Here's the drawing with two shaded views (mm, measured from the low corner). I have some questions. A direction names the side the tool comes from. Give positions to 0.01 mm unless a question says otherwise; leave off trailing zeros. Loops run counter-clockwise (first coordinate to the right, second up) from the corner with the lowest first, then second, coordinate; pieces in that order, holes last. Notation, with made-up numbers: M -2,45.25 L 32,45.25 A18 ccw 32,80.25 Z; hole C 3.25,-13 d5. An arc over 180 degrees is marked long. Write item = value, one per line. Start each with the question number.
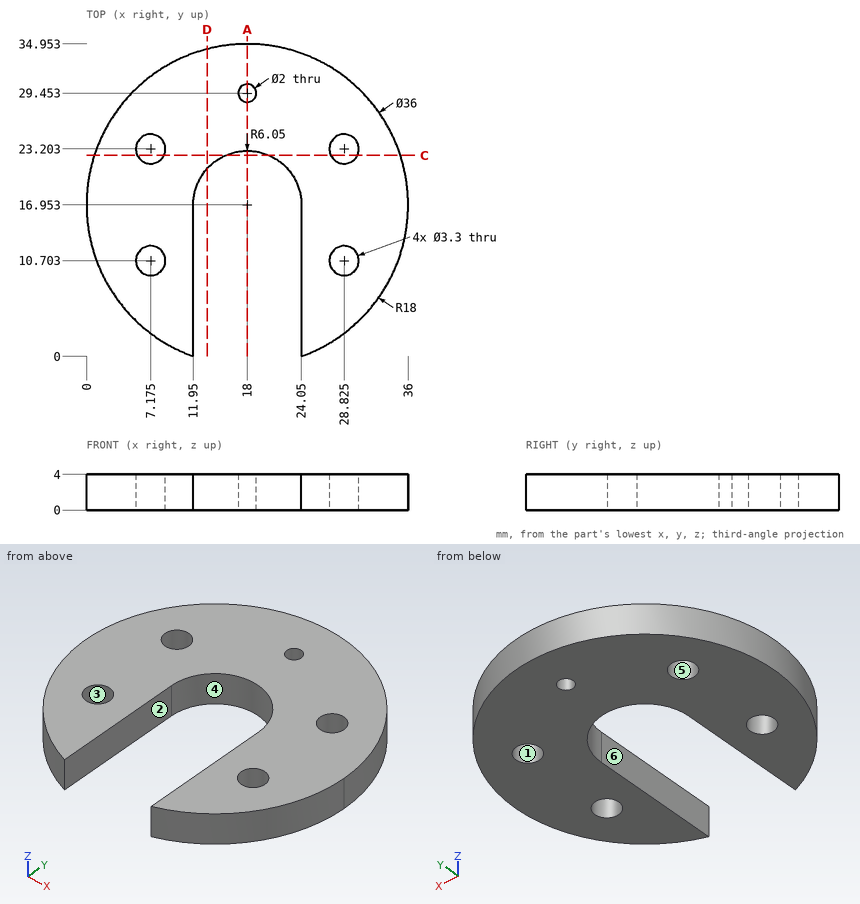
Q1. On a 3-axis mill with a long thin cutter (end or side, diameter ignored), from which of +Z, -Z, +X, -X, +Y, -Y can I reach the whole of each face in a straight line? I mean the marked faces 5 and 6. Say none if no direction works.
Q2. If we section it at D-D, the plane x = 13.5: List the corners of the cut face in (y, z) for me.
Q3. We'd pull the mould along Y, two halves only. Please class the marked faces 1, 2, 3 and 4: pulls with the +Y half, pulls with the -Y half, needs draft (parallel to the pull), parting line crosses it, or undercut.
Q4. If I drill on line 1 along X through (y, z) = (24.5, 1.05) (1 decimal); line 2 along X through (y, z) = (14, 3.35); line 3 along X through (y, z) = (13.5, 3.2), over which ranges is the centre line in solid material (lowest first)?
Q5. If we section it at C-C, the plane y = 22.5: List the corners of the cut face in (x, z) for me (1 decimal).
Q6. If we section it at A-A, the plane x = 18: List the corners of the cut face in (y, z) for me, then the cut area to 3 significant figures.
Q7. Will these pins go through, and if not, where does the flat tip stop? pin 1 (1.5 mm diameter, centred on x = 3.5, z = 1.5, fed in from -Y); pin 2 (4 mm diameter, centred on x = 24, y = 13, fed in from +Z); pin 3 (2 mm diameter, centred on y = 10.5, z = 2, fed in from +X); pin 4 (2.5 mm diameter, centred on x = 7.18, y = 10.7, fed in from +Z).
Resolved:
q1.face_5 = +Z, -Z
q1.face_6 = +Z, -Z, -Y
q2.outline = M 21,0 L 34.38,0 L 34.38,4 L 21,4 Z
q3.face_1 = undercut
q3.face_2 = needs draft
q3.face_3 = undercut
q3.face_4 = pulls with the -Y half
q4.line_1 = 1.7 to 6.2, 8.2 to 27.8, 29.8 to 34.3
q4.line_2 = 0.24 to 11.95, 24.05 to 35.76
q4.line_3 = 0.33 to 11.95, 24.05 to 35.67
q5.outline = M 0.9,0 L 5.7,0 L 5.7,4 L 0.9,4 Z; M 8.7,0 L 15.6,0 L 15.6,4 L 8.7,4 Z; M 20.4,0 L 27.3,0 L 27.3,4 L 20.4,4 Z; M 30.3,0 L 35.1,0 L 35.1,4 L 30.3,4 Z
q6.outline = M 23,0 L 28.45,0 L 28.45,4 L 23,4 Z; M 30.45,0 L 34.95,0 L 34.95,4 L 30.45,4 Z
q6.area = 39.8 mm²
q7.pin_1 = 5.34
q7.pin_2 = 4
q7.pin_3 = 35.15
q7.pin_4 = through
